from build123d import *

# Parameters (mm, degrees)
BOSS_EXTRUDE1_START     = -5
BOSS_EXTRUDE1_OUTLINE_R = 1.925
BOSS_EXTRUDE1_DEPTH     = 5
SKETCH4_R               = 1.6
CUT_EXTRUDE2_DEPTH      = 161.661912101
FILLET1_R               = 15
SKETCH5_R               = 6.5
SKETCH5_R_2             = 2.6
CUT_EXTRUDE4_DEPTH      = 161.661912218
SKETCH6_W               = 233.09675901
SKETCH6_H               = 87.107773224
CUT_EXTRUDE5_DEPTH      = 2


with BuildPart() as part:
    # Boss-Extrude1: read off the stored shape, not the designer's step
    # Boss-Extrude1 outline → Boss-Extrude1 (new body)
    with BuildSketch(Plane.XY.offset(5).offset(BOSS_EXTRUDE1_START)):
        with BuildLine():
            ThreePointArc((149.353851183, 10.916367847), (81.584978704, 16.866619507), (13.564040933, 17.951790818))
            ThreePointArc((13.564040933, 17.951790818), (-22.408339146, -2.028875729), (16.567779435, -15.223622585))
            ThreePointArc((16.567779435, -15.223622585), (81.747231754, -9.530296146), (147.159069574, -10.96780908))
            ThreePointArc((147.159069574, -10.96780908), (158.945093507, -1.097692183), (149.353851183, 10.916367847))
        make_face()
        with Locations((40, 2.5)):
            Circle(BOSS_EXTRUDE1_OUTLINE_R, mode=Mode.SUBTRACT)
        with Locations((95, 2.5)):
            Circle(BOSS_EXTRUDE1_OUTLINE_R, mode=Mode.SUBTRACT)
    extrude(amount=BOSS_EXTRUDE1_DEPTH)

    # Sketch4 → Cut-Extrude2 (cut, through all)
    with BuildSketch(Plane.XY.offset(5)):
        with Locations((0, 17)):
            Circle(SKETCH4_R)
        with Locations((16.167960777, 5.253288904)):
            Circle(SKETCH4_R)
        with Locations((9.992349289, -13.753288904)):
            Circle(SKETCH4_R)
        with Locations((-9.992349289, -13.753288904)):
            Circle(SKETCH4_R)
        with Locations((-16.167960777, 5.253288904)):
            Circle(SKETCH4_R)
    extrude(amount=-CUT_EXTRUDE2_DEPTH, mode=Mode.SUBTRACT)

    # Fillet1
    fillet1_edges = [part.edges().sort_by_distance(p)[0] for p in [
        (16.567779435, -15.223622585, 2.5),
        (13.564040933, 17.951790818, 2.5),
    ]]
    fillet(fillet1_edges, radius=FILLET1_R)

    # Sketch5 → Cut-Extrude4 (cut, through all)
    with BuildSketch(Plane.XY.offset(5)):
        Circle(SKETCH5_R)
        with Locations((148, 0)):
            Circle(SKETCH5_R_2)
        with Locations((95, 2.5)):
            Circle(SKETCH5_R_2)
        with Locations((40, 2.5)):
            Circle(SKETCH5_R_2)
    extrude(amount=-CUT_EXTRUDE4_DEPTH, mode=Mode.SUBTRACT)

    # Sketch6 → Cut-Extrude5 (cut)
    with BuildSketch(Plane.XY.offset(5)):
        with Locations((68.481602645, 0)):
            Rectangle(SKETCH6_W, SKETCH6_H)
    extrude(amount=-CUT_EXTRUDE5_DEPTH, mode=Mode.SUBTRACT)


solid = part.part
Geometry check sheet. Reference: the model listing, model coordinates, mm. Coordinates: 2 decimals unless noted, no trailing zeros. Loops run counter-clockwise (first coordinate to the right, second up) from the corner with the lowest first, then second, coordinate; pieces in that order, holes last. Notation, with made-up numbers: (67.25, -12) - (81.25, -12) arc R28 cw to (81.25, 14) - close; hole circle Ø9 at (-23.75, -31). An arc over 180 degrees is marked (long way). Use one line per item in the form item = value. Start each with the question number.
Item 1: Section check B-B, the plane y = -5. Enter the section's corners in (x, z), and give its area (3 significant figures).
Item 2: Section check D-D, the plane y = 9. Enter the section's corners in (x, z), and give its area (3 significant figures).
Item 3: Gauge pin test, flat ends, axial feed: pin 1 (1.5 mm diameter, centred on y = 9.5, z = 2, fed in from +X); pin 2 (4.5 mm diameter, centred on x = 148, y = 0, fed in from +Z); pin 3 (1 mm diameter, centred on y = 14, z = 1, fed in from -X). Record the tip position at first contact, or that the pin passes through.
Item 4: Mould release check, pull along X, two halves, no side actions. Record for faces 1 (the face through (-22.463, -1.284, 1.479)), 2 (the face through (47, 0, 3)), 3 (the face through (83.212, -9.484, 1.479)): +X half, -X half, draft (parallel to the pull), parting line (faces both ways), or undercut.
Item 5: Section check A-A, the plane x = 0. Enter the section's corners in (y, z).
Item 6: Thickness scan on probe 1 along Y at (x, z) = (0, 1.35); probe 2 along X at (y, z) = (-1, 2.55); probe 3 along X at (y, z) = (6, 0.4). Record the ranges inside material, lowest first.
Item 7: Section check C-C, the plane x = 95. Enter the section's corners in (y, z).
Computed:
q1.outline = (-21.94, 0) - (-4.15, 0) - (-4.15, 3) - (-21.94, 3) - close; (4.15, 0) - (157.8, 0) - (157.8, 3) - (4.15, 3) - close
q1.area = 514 mm2
q2.outline = (-20.62, 0) - (154.32, 0) - (154.32, 3) - (-20.62, 3) - close
q2.area = 525 mm2
q3.pin_1 = 154.67
q3.pin_2 = through
q3.pin_3 = -18
q4.face_1 = parting line
q4.face_2 = draft
q4.face_3 = undercut
q5.outline = (-22.5, 0) - (-6.5, 0) - (-6.5, 3) - (-22.5, 3) - close; (6.5, 0) - (15.4, 0) - (15.4, 3) - (6.5, 3) - close; (18.6, 0) - (22.5, 0) - (22.5, 3) - (18.6, 3) - close
q6.probe_1 = -22.5 to -6.5, 6.5 to 15.4, 18.6 to 22.5
q6.probe_2 = -22.48 to -6.42, 6.42 to 145.6, 150.4 to 158.95
q6.probe_3 = -21.69 to -17.58, -14.75 to -2.5, 2.5 to 14.75, 17.58 to 157.22
q7.outline = (-9.24, 0) - (-0.1, 0) - (-0.1, 3) - (-9.24, 3) - close; (5.1, 0) - (16.08, 0) - (16.08, 3) - (5.1, 3) - close
